Here's how the part is built. I have some questions about the finished solid (model axes, mm). A direction names the side the tool comes from. Coordinates: 2 decimals unless noted, no trailing zeros. Write each loop counter-clockwise with the first axis right and the second up, starting at its lowest first coordinate (ties: lowest second). Pieces come first, ordered by that corner, then holes.
Item 1: I'm going to push flat-ended pins straight in: pin 1 Ø6 at (y, z) = (7.5, 2) entering from -X; pin 2 Ø1 at (x, z) = (0, -9) entering from +Y; pin 3 Ø1 at (x, y) = (7, 2.5) entering from +Z; pin 4 Ø2 at (y, z) = (8, 1.5) entering from -X. Where does each tip first touch, or does it pass through?
Item 2: If I drill on line 1 (X direction, y = -2.5, z = 0.25); line 2 (Y direction, x = 2, z = -8.25); line 3 (Z direction, x = -3.75, y = -1), over which ranges is the centre line in solid material (lowest first)?
Item 3: We'd pull the mould along Z, two halves only. Please class faces 4 (the face through (-8, 9, 4)), 5 (the face through (7.412, 8.014, 5.145)), 6 (the face through (2.603, 8.014, 8.639)): +Z half, -Z half, draft (parallel to the pull), parting line (faces both ways), or undercut.
Item 4: If we section it at A-A (y = -0.5): Please give me the cut outline in (x, z), then the cut area to 3 significant figures.
Item 5: If we section it at B-B (y = 2.75): Please give me the cut outline in (x, z), then the cut area to 3 significant figures.
Item 6: For faces 1 (the face through (7, 7, -6)), 2 (the face through (2, 9, 9)), 3 (the face through (-5, 7.65, -7)), which set-ups out of +Z, -Z, +X, -X, +Y, -Y let a thin tool reach every point of the face, with its end or its side?
from build123d import *

# Parameters (mm, degrees)
SKETCH1_R           = 6.5
BOSS_EXTRUDE1_DEPTH = 8
BOSS_EXTRUDE1_DRAFT = -14
SKETCH2_R           = 6.2
BOSS_EXTRUDE2_DEPTH = 5
SKETCH3_R           = 5.75
CUT_EXTRUDE1_DEPTH  = 5
SKETCH5_W           = 0.7
SKETCH5_H           = 0.7
SKETCH6_W           = 1.273218484
SKETCH6_H           = 2
BOSS_EXTRUDE4_DEPTH = 0.75
CIRPATTERN1_COUNT   = 15


with BuildPart() as part:
    # Sketch1 → Boss-Extrude1 (with draft: the straight prism first)
    with BuildSketch(Plane(origin=(0, 0, 0), x_dir=(1, 0, 0), z_dir=(0, 1, 0))):
        Circle(SKETCH1_R)
    extrude(amount=BOSS_EXTRUDE1_DEPTH)
    # Boss-Extrude1: the draft: its side faces are tilted about the plane it starts from
    boss_extrude1_sides = [part.faces().sort_by_distance(p)[0] for p in [
        (-6.5, 4, 0),
    ]]
    draft(boss_extrude1_sides, Plane(origin=(0, 0, 0), x_dir=(1, 0, 0), z_dir=(0, 1, 0)), BOSS_EXTRUDE1_DRAFT)

    # Sketch2 → Boss-Extrude2 (add)
    with BuildSketch(Plane.XZ):
        with Locations(Location((0, 0, 0), (0, 0, 270))):
            Circle(SKETCH2_R)
    extrude(amount=BOSS_EXTRUDE2_DEPTH)

    # Sketch3 → Cut-Extrude1 (cut)
    with BuildSketch(Plane.XZ.offset(5)):
        with Locations(Location((0, 0, 0), (0, 0, 270))):
            Circle(SKETCH3_R)
    extrude(amount=-CUT_EXTRUDE1_DEPTH, mode=Mode.SUBTRACT)

    # Sketch4 → Revolve1 (revolve)
    with BuildSketch(Plane(origin=(0, 0, 0), x_dir=(0, 0, -1), z_dir=(1, 0, 0)), mode=Mode.PRIVATE) as revolve1_sk:
        with BuildLine():
            Line((0, 8), (0, 10.5))
            add(Edge.make_bspline(
                [(0, 10.5), (4.616560174, 10.68965763), (8.494624023, 8)],
                knots=[0, 0, 0, 1, 1, 1], degree=2))
            Line((8.494624023, 8), (0, 8))
        make_face()
    revolve(revolve1_sk.sketch.rotate(Axis((0, 8, 0), (0, 1, 0)), 180), axis=Axis((0, 8, 0), (0, 1, 0)))

    # Sketch5 → Revolve2 (revolve)
    with BuildSketch(Plane(origin=(0, 0, 0), x_dir=(0, 0, -1), z_dir=(1, 0, 0))):
        with Locations((8.494624023, 8)):
            Rectangle(SKETCH5_W, SKETCH5_H)
    revolve(axis=Axis((0, -5.748475936, 0), (0, 1, 0)))

    # Sketch6 → Boss-Extrude4 (add, symmetric)
    with BuildSketch(Plane(origin=(0, 0, 0), x_dir=(0, 0, -1), z_dir=(1, 0, 0))):
        with Locations((9, 8)):
            Rectangle(SKETCH6_W, SKETCH6_H)
    boss_extrude4 = extrude(amount=BOSS_EXTRUDE4_DEPTH, both=True)

    # CirPattern1: Boss-Extrude4 ×15 about axis
    cirpattern1_axis = Axis((0, 0, 0), (0, 1, 0))
    for i in range(1, CIRPATTERN1_COUNT):
        add(boss_extrude4.rotate(cirpattern1_axis, i * 360 / CIRPATTERN1_COUNT))


solid = part.part
Answer list:
1. pin 1: stops at x = -9.66
1. pin 2: stops at y = 9
1. pin 3: stops at z = 2.95
1. pin 4: stops at x = -9.64
2. line 1: x = -6.19 to -5.74, 5.74 to 6.19
2. line 2: y = 7.65 to 8.35
2. line 3: z = -4.94 to -4.36, 4.36 to 4.94
3. face 4: draft
3. face 5: +Z half
3. face 6: undercut
4. outline: circle Ø12.4 at (0, 0); hole circle Ø11.5 at (0, 0)
4. area: 16.9 mm2
5. outline: circle Ø14.37 at (0, 0)
5. area: 162 mm2
6. face 1: -Z, +X, -Y
6. face 2: +Z, +X, -X, +Y
6. face 3: -Y
